Model file for the job. Use its own axes, mm. Round coordinates to 2 decimals unless told otherwise and drop trailing zeros. Order: outer loops, then holes, each group sorted by start corner. A loop starts at its lowest first (then second) coordinate and runs counter-clockwise, first axis right, second up. Notation, with made-up numbers: (74.25, 49) - (96.25, 49) arc R10 cw to (96.25, 56) - close; hole circle Ø9 at (27.5, -32). An arc over 180 degrees is marked (long way). Put each result on its own line as item: value. Start each with the question number.
Item 1: Pin check, flat tips, straight feed: pin 1 Ø3 at (x, z) = (-3, -63) entering from +Y; pin 2 Ø4 at (x, y) = (0, 0) entering from +Z; pin 3 Ø4 at (x, z) = (3, 10.5) entering from -Y. Stop position of each tip, or through.
Item 2: Saw through at A-A on y = 0. List the corners of the cut face in (x, z) (3 decimals).
Item 3: Mould opens along Y. For faces 1 (the face through (-3.21, 5.48, -1.11)), 2 (the face through (6.35, 0, -1)), 3 (the face through (-0.767, -2.435, -1.111)) say: pulls with the +Y half, pulls with the -Y half, needs draft (parallel to the pull), parting line crosses it, or undercut.
Item 4: Saw through at B-B on z = 55.5. List the corners of the cut face in (x, y), plus the area to 3 significant figures.
Item 5: Probe probe 1 along X at (y, z) = (0, 11); probe 2 along Y at (x, z) = (0, 33); probe 3 along X at (y, z) = (0.5, -36). List the from-to ranges inside material, lowest first.
Autodesk Inventor part; units mm, degrees
ref_plane "YZ Plane" through (0, 0, 0) normal (1, 0, 0) x (0, 1, 0)
ref_plane "XZ Plane" through (0, 0, 0) normal (0, 1, 0) x (-1, 0, 0)
ref_plane "XY Plane" through (0, 0, 0) normal (0, 0, 1) x (1, 0, 0)
sketch "Sketch1" plane through (0, 0, 0) normal (0, 0, 1) x (1, 0, 0)
  line L0 (-6.35, -3.6662) -> (-6.35, 3.6662)
  line L1 (-6.35, 3.6662) -> (0, 7.3323)
  line L2 (0, 7.3323) -> (6.35, 3.6662)
  line L3 (6.35, 3.6662) -> (6.35, -3.6662)
  line L4 (6.35, -3.6662) -> (0, -7.3323)
  line L5 (0, -7.3323) -> (-6.35, -3.6662)
  point P0 (0, 0)
  point P1 (0, 0)
  dimension "Size" = 12.7
extrude "Extrusion1" add sketch "Sketch1" along normal mid plane 158.75
sketch "Sketch3" plane through (0, 0, 79.375) normal (0, 0, 1) x (1, 0, 0)
  line L0 (-6.35, 3.6662) -> (0, 7.3323) construction
  line L1 (0, 7.3323) -> (6.35, 3.6662) construction
  line L2 (6.35, 3.6662) -> (6.35, -3.6662) construction
  line L3 (6.35, -3.6662) -> (0, -7.3323) construction
  line L4 (0, -7.3323) -> (-6.35, -3.6662) construction
  line L5 (-6.35, -3.6662) -> (-6.35, 3.6662) construction
  point P0 (0, 0)
hole "Hole1" at (0, 0, 79.375) direction (0, 0, -1) diameter 5.1054 end through all
sketch "Sketch4" plane through (0, 0, 79.375) normal (0, 0, 1) x (1, 0, 0)
  circle A0 centre (0, 0) radius 2.5527 construction
  line L0 (-6.35, 3.6662) -> (0, 7.3323) construction
  line L1 (0, 7.3323) -> (6.35, 3.6662) construction
  line L2 (6.35, 3.6662) -> (6.35, -3.6662) construction
  line L3 (6.35, -3.6662) -> (0, -7.3323) construction
  line L4 (0, -7.3323) -> (-6.35, -3.6662) construction
  line L5 (-6.35, -3.6662) -> (-6.35, 3.6662) construction
  circle A1 centre (0, 0) radius 6.8771
  circle A2 centre (0, 0) radius 8.89
  dimension "thunder" = 13.7541
  dimension "d16" = 17.78
extrude "Extrusion3" cut sketch "Sketch4" against normal through all
equation "\"bearing\" = 25.4"
properties part number "GP5-010" material "Aluminum 6061"
Results found:
1. pin 1: stops at y = 6.47
1. pin 2: passes through
1. pin 3: stops at y = -6.75
2. outline: (-6.35, -79.375) - (-2.553, -79.375) - (-2.553, 79.375) - (-6.35, 79.375) - close; (2.553, -79.375) - (6.35, -79.375) - (6.35, 79.375) - (2.553, 79.375) - close
3. face 1: pulls with the +Y half
3. face 2: needs draft
3. face 3: undercut
4. outline: (-6.35, -2.64) arc R6.88 ccw to (-5.46, -4.18) - (-0.89, -6.82) arc R6.88 ccw to (0.89, -6.82) - (5.46, -4.18) arc R6.88 ccw to (6.35, -2.64) - (6.35, 2.64) arc R6.88 ccw to (5.46, 4.18) - (0.89, 6.82) arc R6.88 ccw to (-0.89, 6.82) - (-5.46, 4.18) arc R6.88 ccw to (-6.35, 2.64) - close; hole circle Ø5.11 at (0, 0)
4. area: 117 mm²
5. probe 1: x = -6.35 to -2.55, 2.55 to 6.35
5. probe 2: y = -6.88 to -2.55, 2.55 to 6.88
5. probe 3: x = -6.35 to -2.5, 2.5 to 6.35
